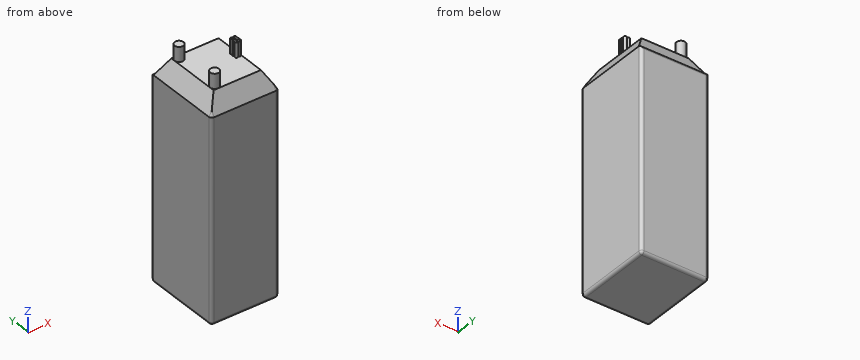
Autodesk Inventor part; units mm, degrees
ref_plane "YZ Plane" through (0, 0, 0) normal (1, 0, 0) x (0, 1, 0)
ref_plane "XZ Plane" through (0, 0, 0) normal (0, 1, 0) x (-1, 0, 0)
ref_plane "XY Plane" through (0, 0, 0) normal (0, 0, 1) x (1, 0, 0)
sketch "Sketch1" plane through (0, 0, 0) normal (0, 0, 1) x (1, 0, 0)
  line L0 (-23, 27) -> (23, 27)
  line L1 (23, 27) -> (23, -27)
  line L2 (23, -27) -> (-23, -27)
  line L3 (-23, -27) -> (-23, 27)
  line L4 (-23, 27) -> (23, -27) construction
  line L5 (23, 27) -> (-23, -27) construction
  point P0 (0, 0)
  dimension "d0" = 46
  dimension "d1" = 54
extrude "Extrusion1" add sketch "Sketch1" along normal blind 137
fillet "Fillet1" radius 2 9 edges at (-23, 27, 68.5) (0, 27, 137) (23, 27, 68.5) (0, 27, 0) (23, -27, 68.5) (23, 0, 0) (-23, 0, 0) (-23, -27, 68.5) (0, -27, 0)
sketch "Sketch2" plane through (-23, 27, 0) normal (0, 1, 0) x (1, 0, 0)
  line L0 (2, -131.2678) -> (2, -4.2112) construction
  line L1 (2, -4.2112) -> (44, -4.2112) construction
  line L2 (44, -4.2112) -> (44, -131.2678) construction
  line L3 (44, -131.2678) -> (2, -131.2678) construction
  line L4 (2, -135) -> (2, -2)
  line L5 (44, -2) -> (44, -135)
  point P0 (23, 0)
sketch "Sketch3" plane through (0, 0, 137) normal (0, 0, 1) x (1, 0, 0)
  arc A0 (-23, -25) -> (-21, -27) centre (-21, -25) ccw
  line L0 (-21, -27) -> (21, -27)
  arc A1 (21, -27) -> (23, -25) centre (21, -25) ccw
  line L1 (23, -25) -> (23, 25)
  line L2 (-23, 25) -> (23, 25)
  line L3 (-23, 25) -> (-23, -25)
  point P0 (0, 0)
extrude "Extrusion2" add sketch "Sketch3" along normal blind 12 draft -30
sketch "Sketch4" plane through (0, 0, 149) normal (0, 0, 1) x (1, 0, 0)
  circle A0 centre (-13.0718, 15.0718) radius 3
  circle A1 centre (-13.0718, -17.0718) radius 3
  line L0 (-16.0718, 18.0718) -> (16.0718, 18.0718)
  line L1 (-16.0718, -20.0718) -> (-16.0718, 18.0718)
  line L2 (16.0718, 18.0718) -> (16.0718, -20.0718)
  circle A2 centre (13.0718, 0) radius 1
  circle A3 centre (15.0718, 0) radius 1
  circle A4 centre (15.0718, 2) radius 1
  circle A5 centre (13.0718, 2) radius 1
  line L3 (16.0718, -20.0718) -> (-16.0718, -20.0718)
  circle A6 centre (13.0718, -2) radius 1
  circle A7 centre (15.0718, -2) radius 1
  line L4 (0, 0) -> (13.0718, 0) construction
  point P0 (13.0718, 1)
  point P1 (14.0718, 2)
  point P2 (15.0718, 1)
  point P3 (14.0718, 0)
  point P4 (14.0718, -2)
  dimension "d45" = 6
  dimension "d46" = 6
  dimension "d48" = 2
extrude "Extrusion3" add sketch "Sketch4" along normal blind 10 contours A0 | A1 | A4 | A3 | A5 | A7 | A2 | A6
properties part number "Lipo Battery CNHL 4000mAh"
Geometry: final body of the model. Coordinates: model frame, mm. Coordinates: 2 decimals unless noted, no trailing zeros. Order: outer loops, then holes, each group sorted by start corner. A loop starts at its lowest first (then second) coordinate and runs counter-clockwise, first axis right, second up.
1) First-contact query: P1, Ø9.5, axis at x = 0.5, y = -3, coming from the +Z side. Flat tip, straight axial feed; report the tip coordinate or a pass-through.
Result sheet:
P1: stops at z = 149
2) Section A-A (y = -12.5). Return loops of the section in (x, z).
Result sheet:
outline: (-23, 2) arc R2 ccw to (-21, 0) - (21, 0) arc R2 ccw to (23, 2) - (23, 137) - (16.07, 149) - (-16.07, 149) - (-23, 137) - close
3) Ray query, probe 1 along Z at (x, y) = (-8.5, -2.5); probe 2 along Z at (x, y) = (2, -23). Return the intervals inside material, ascending.
Result sheet:
probe 1: z = 0 to 149
probe 2: z = 0 to 143.93
4) Section B-B (x = -1). Return loops of the section in (y, z).
Result sheet:
outline: (-27, 2) arc R2 ccw to (-25, 0) - (25, 0) arc R2 ccw to (27, 2) - (27, 135) arc R2 ccw to (25, 137) - (18.07, 149) - (-20.07, 149) - (-27, 137) - close
5) Section C-C (x = 19). Return loops of the section in (y, z), then the cut area to 3 significant figures.
Result sheet:
outline: (-27, 2) arc R2 ccw to (-25, 0) - (25, 0) arc R2 ccw to (27, 2) - (27, 135) arc R2 ccw to (25, 137) - (21, 143.93) - (-23, 143.93) - (-27, 137) - close
area: 7,730 mm2
